Autodesk Inventor part; units mm, degrees
ref_plane "YZ Plane" through (0, 0, 0) normal (1, 0, 0) x (0, 1, 0)
ref_plane "XZ Plane" through (0, 0, 0) normal (0, 1, 0) x (-1, 0, 0)
ref_plane "XY Plane" through (0, 0, 0) normal (0, 0, 1) x (1, 0, 0)
sketch "Sketch1" plane through (0, 0, 0) normal (0, 1, 0) x (-1, 0, 0)
  line L0 (9.1654, 15.875) -> (18.3309, 0)
  line L1 (18.3309, 0) -> (9.1654, -15.875)
  line L2 (9.1654, -15.875) -> (-9.1654, -15.875)
  line L3 (-9.1654, -15.875) -> (-18.3309, 0)
  line L4 (-18.3309, 0) -> (-9.1654, 15.875)
  line L5 (-9.1654, 15.875) -> (9.1654, 15.875)
  point P0 (0, 0)
  point P1 (0, 0)
  dimension "HEX_FLATS" = 31.75
extrude "Extrusion1" add sketch "Sketch1" along normal blind 13.3096
sketch "Sketch2" plane through (0, 0, 0) normal (0, 0, 1) x (1, 0, 0)
  line L0 (9.1654, 13.3096) -> (18.3309, 13.3096)
  line L1 (15.875, 13.3096) -> (28.575, 5.9773)
  line L2 (28.575, 5.9773) -> (28.575, 18.6773)
  line L3 (28.575, 18.6773) -> (15.875, 18.6773)
  line L4 (15.875, 18.6773) -> (15.875, 13.3096)
  line L5 (0, 26.9922) -> (0, -31.2125)
  line L6 (0, 0) -> (0, -22.8975)
  dimension "d3" = 30
  dimension "HD_CHAMFER" = 15.875
  dimension "d5" = 12.7
  dimension "d6" = 12.7
revolve "Revolution1" cut sketch "Sketch2" angle 360 about axis through (0, 0, 0) along (0, -1, 0)
sketch "Sketch3" plane through (0, 0, 0) normal (0, -1, 0) x (1, 0, 0)
  circle A0 centre (0, 0) radius 7.5
  dimension "BOLT_SIZE" = 15
extrude "Extrusion2" add sketch "Sketch3" along normal blind 76.2
chamfer "Chamfer1" distance 1.524 angle 45 1 edges at (-7.5, -76.2, 0)
thread "Thread 1/2\""
thread "Thread 5/8\""
thread "Thread-3/4\""
thread "Thread 7/8\""
thread "Thread 1\""
thread "Thread 1 1/8\""
thread "Thread 1 1/4\""
properties material "Stainless Steel"
Design review of the part built by this model. Coordinates are the model's own, in mm. A direction names the side the tool comes from. Coordinates: 2 decimals unless noted, no trailing zeros. Order: outer loops, then holes, each group sorted by start corner. A loop starts at its lowest first (then second) coordinate and runs counter-clockwise, first axis right, second up. Notation, with made-up numbers: M 66,0.5 L 99,0.5 A27 cw 99,25.5 Z; hole C 6.5,56 d3. An arc over 180 degrees is marked long. Answer as a JSON object with one key per item and string values. Group by question number.
1) Tool access review of faces 1 (the flat face through (-8, 0, 0)), 2 (the flat face through (-13.684, 6.562, 8.049)): name each direction out of +Z, -Z, +X, -X, +Y, -Y from which nothing blocks a thin tool from reaching the whole face with its end or side.
2) Add section B-B, the plane y = -67.5. Write out the cut boundary in (x, z).
3) Wall thickness on L1, parallel to Y at x = 9, z = 11; L2, parallel to Z at x = -0.5, y = -62; L3, parallel to Z at x = 2.5, y = -55: over which ranges is each line inside the solid? List them lowest first.
4) Add section A-A, the plane y = 6. Write out the cut boundary in (x, z) (3 decimals), then the cut area to 3 significant figures.
5) For pin 1 (1 mm diameter, centred on x = -8, z = 9, fed in from -Y); pin 2 (6 mm diameter, centred on x = -3, y = -23, fed in from -Z); pin 3 (1 mm diameter, centred on x = 3.5, y = -20.5, fed in from +Z); pin 4 (2 mm diameter, centred on x = -9.5, y = -2.5, fed in from -Z), all flat-tipped, find the tip position at first contact; note any pin that passes through.
Computed values:
{
 "1": {"face 1": "-Y", "face 2": "+Z, -X, +Y, -Y"},
 "2": {"outline": "C 0,0 d15"},
 "3": {"L1": "y = 0 to 13.31", "L2": "z = -7.48 to 7.48", "L3": "z = -7.07 to 7.07"},
 "4": {"outline": "M -18.331,0 L -9.165,-15.875 L 9.165,-15.875 L 18.331,0 L 9.165,15.875 L -9.165,15.875 Z", "area": "873 mm^2"},
 "5": {"pin 1": "stops at y = 0", "pin 2": "stops at z = -7.5", "pin 3": "stops at z = 6.87", "pin 4": "passes through"}
}
